Check sheet for the modelled part. Datum: model origin and axes. Units: mm. A direction names the side the tool comes from. Round coordinates to 2 decimals unless told otherwise and drop trailing zeros. Loops run counter-clockwise (first coordinate to the right, second up) from the corner with the lowest first, then second, coordinate; pieces in that order, holes last. Notation, with made-up numbers: (-28.5, 63) - (-16.5, 63) arc R17 ccw to (-16.5, 90) - close; hole circle Ø1 at (6, 21.5). An arc over 180 degrees is marked (long way). Answer in a Markdown table with one row per item. Add a question column.
(1) Mould release check, pull along X, two halves, no side actions. Record for faces 1 (the flat face through (-2, 25.4, 2)), 2 (the flat face through (-244.475, 0, -60)), 3 (the flat face through (-2, -25.4, 2)), 4 (the flat face through (170, -31.75, -55)): +X half, -X half, draft (parallel to the pull), parting line (faces both ways), or undercut.
(2) Access from +Z, -Z, +X, -X, +Y, -Y to the whole of each face (thin tool, end or side, straight path). Record for faces 5 (the flat face through (-15, 0, 0)), 6 (the flat face through (-218, 0, -44.45)), 7 (the flat face through (175, 0, -76.2)), 8 (the flat face through (218, 0, -44.45)), 9 (the flat face through (1, 0, 50.8)).
(3) Cross-section at B-B on z = -20. Enter the section's corners in (x, y), then the cut area to 3 significant figures.
(4) Gauge pin test, flat ends, axial feed: pin 1 (5 mm diameter, centred on y = -16, z = 14.5, fed in from +X); pin 2 (15 mm diameter, centred on x = -8.5, y = 4.5, fed in from -Z); pin 3 (1 mm diameter, centred on y = 17, z = -9.5, fed in from -X). Record the tip position at first contact, or that the pin passes through.
(5) Cross-section at A-A on y = 20. Enter the section's corners in (x, z) (3 decimals).
(6) Cross-section at D-D on y = -6. Enter the section's corners in (x, z) (3 decimals).
(7) Thickness scan on line 1 along Z through (x, y) = (203, 20.5); line 2 along Y through (x, z) = (-83, -32). Record the ranges inside material, lowest first.
(8) Cross-section at C-C on x = 204. Enter the section's corners in (y, z).
from build123d import *

# Parameters (mm, degrees)
F1_DEPTH     = 25.4
F2_DEPTH     = 31.75
F3_T4_DEPTH  = 86.0090909091
F3_T9_DEPTH  = 86.0090909091
F3_T14_DEPTH = 86.0090909091
F3_T19_DEPTH = 86.0090909091
F3_T21_DEPTH = 93.5090909091


# Not quite as in the source:
# - a fillet or chamfer that OpenCascade refuses, or shapes differently, is made with other operations: its cross-section is extruded or revolved along the edge and cut away or added


with BuildPart() as f1:
    # F0 (on Front) → F1 (new body, symmetric)
    with BuildSketch(Plane.XZ):
        with BuildLine():
            Line((-107.95, -76.2), (-63.0464285714, 0))
            Line((-63.0464285714, 0), (0, 0))
            Line((0, 0), (0, 9.525))
            ThreePointArc((0, 9.525), (8.6950956004, 6.9319779212), (14.5496778315, 0))
            Line((14.5496778315, 0), (63.0464285714, 0))
            Line((63.0464285714, 0), (107.95, -76.2))
            Line((107.95, -76.2), (120.65, -76.2))
            Line((120.65, -76.2), (120.65, 2.3090909091))
            Line((120.65, 2.3090909091), (92.075, 50.8))
            Line((92.075, 50.8), (-92.075, 50.8))
            Line((-92.075, 50.8), (-120.65, 2.3090909091))
            Line((-120.65, 2.3090909091), (-120.65, -76.2))
            Line((-120.65, -76.2), (-107.95, -76.2))
        make_face()
        with BuildLine():
            Line((0, 9.525), (0, 0))
            Line((0, 0), (14.5496778315, 0))
            ThreePointArc((14.5496778315, 0), (8.6950956004, 6.9319779212), (0, 9.525))
        make_face()
    extrude(amount=F1_DEPTH, both=True)

    # F0 (on Front) → F2 (join, symmetric)
    with BuildSketch(Plane.XZ):
        with BuildLine():
            Line((-244.475, -76.2), (-120.65, -76.2))
            Line((-120.65, -76.2), (-120.65, 2.3090909091))
            Line((-120.65, 2.3090909091), (-126.0980906593, -6.9361538462))
            ThreePointArc((-126.0980906593, -6.9361538462), (-153.9415343258, -34.4101274299), (-191.7473214286, -44.45))
            Line((-191.7473214286, -44.45), (-244.475, -44.45))
            Line((-244.475, -44.45), (-244.475, -76.2))
        make_face()
        with BuildLine():
            Line((120.65, 2.3090909091), (120.65, -76.2))
            Line((120.65, -76.2), (244.475, -76.2))
            Line((244.475, -76.2), (244.475, -44.45))
            Line((244.475, -44.45), (191.7473214286, -44.45))
            ThreePointArc((191.7473214286, -44.45), (153.9415343258, -34.4101274299), (126.0980906593, -6.9361538462))
            Line((126.0980906593, -6.9361538462), (120.65, 2.3090909091))
        make_face()
    extrude(amount=F2_DEPTH, both=True)

    # F3: fillet of radius 3 on 8 edges, made by hand


with BuildPart() as f3_tool2:
    # F3_s3 → F3_t4 (new body)
    with BuildSketch(Plane.XY.offset(9.8090909091)):
        with BuildLine():
            ThreePointArc((-120.65, -28.4), (-119.7713203436, -26.2786796564), (-117.65, -25.4))
            Line((-117.65, -25.4), (-120.65, -25.4))
            Line((-120.65, -25.4), (-120.65, -28.4))
        make_face()
    extrude(amount=-F3_T4_DEPTH)

    split(bisect_by=Plane(origin=(-90.5622721893, 0, 53.3670532544), x_dir=(0, 1, 0), z_dir=(0.8615384615, 0, -0.5076923077)), keep=Keep.TOP)


with BuildPart() as f1_1:
    add(f1.part)

    # F3_t1: union F3_tool2
    add(f3_tool2.part)


with BuildPart() as f3_tool7:
    # F3_s8 → F3_t9 (new body)
    with BuildSketch(Plane.XY.offset(9.8090909091)):
        with BuildLine():
            ThreePointArc((-120.65, 28.4), (-119.7713203436, 26.2786796564), (-117.65, 25.4))
            Line((-117.65, 25.4), (-120.65, 25.4))
            Line((-120.65, 25.4), (-120.65, 28.4))
        make_face()
    extrude(amount=-F3_T9_DEPTH)

    split(bisect_by=Plane(origin=(-90.5622721893, 0, 53.3670532544), x_dir=(0, 1, 0), z_dir=(0.8615384615, 0, -0.5076923077)), keep=Keep.TOP)


with BuildPart() as f1_2:
    add(f1_1.part)

    # F3_t6: union F3_tool7
    add(f3_tool7.part)


with BuildPart() as f3_tool12:
    # F3_s13 → F3_t14 (new body)
    with BuildSketch(Plane.XY.offset(-76.2)):
        with BuildLine():
            ThreePointArc((117.65, 25.4), (119.7713203436, 26.2786796564), (120.65, 28.4))
            Line((120.65, 28.4), (120.65, 25.4))
            Line((120.65, 25.4), (117.65, 25.4))
        make_face()
    extrude(amount=F3_T14_DEPTH)

    split(bisect_by=Plane(origin=(90.5622721893, 0, 53.3670532544), x_dir=(0, 1, 0), z_dir=(-0.8615384615, 0, -0.5076923077)), keep=Keep.TOP)


with BuildPart() as f1_3:
    add(f1_2.part)

    # F3_t11: union F3_tool12
    add(f3_tool12.part)


with BuildPart() as f3_tool17:
    # F3_s18 → F3_t19 (new body)
    with BuildSketch(Plane.XY.offset(-76.2)):
        with BuildLine():
            ThreePointArc((117.65, -25.4), (119.7713203436, -26.2786796564), (120.65, -28.4))
            Line((120.65, -28.4), (120.65, -25.4))
            Line((120.65, -25.4), (117.65, -25.4))
        make_face()
    extrude(amount=F3_T19_DEPTH)

    split(bisect_by=Plane(origin=(90.5622721893, 0, 53.3670532544), x_dir=(0, 1, 0), z_dir=(-0.8615384615, 0, -0.5076923077)), keep=Keep.TOP)


with BuildPart() as f1_4:
    add(f1_3.part)

    # F3_t16: union F3_tool17
    add(f3_tool17.part)

    # F3_s22 → F3_t21 (cut)
    with BuildSketch(Plane.XY.offset(-83.7)):
        with BuildLine():
            ThreePointArc((-120.65, -28.75), (-121.5286796564, -30.8713203436), (-123.65, -31.75))
            Line((-123.65, -31.75), (-120.65, -31.75))
            Line((-120.65, -31.75), (-120.65, -28.75))
        make_face()
        with BuildLine():
            ThreePointArc((-123.65, 31.75), (-121.5286796564, 30.8713203436), (-120.65, 28.75))
            Line((-120.65, 28.75), (-120.65, 31.75))
            Line((-120.65, 31.75), (-123.65, 31.75))
        make_face()
        with BuildLine():
            ThreePointArc((120.65, 28.75), (121.5286796564, 30.8713203436), (123.65, 31.75))
            Line((123.65, 31.75), (120.65, 31.75))
            Line((120.65, 31.75), (120.65, 28.75))
        make_face()
        with BuildLine():
            ThreePointArc((123.65, -31.75), (121.5286796564, -30.8713203436), (120.65, -28.75))
            Line((120.65, -28.75), (120.65, -31.75))
            Line((120.65, -31.75), (123.65, -31.75))
        make_face()
    extrude(amount=F3_T21_DEPTH, mode=Mode.SUBTRACT)

    # F0 (on Front) → F4 (revolve, cut)
    with BuildSketch(Plane.XZ):
        with BuildLine():
            Line((0, 9.525), (0, 0))
            Line((0, 0), (14.5496778315, 0))
            ThreePointArc((14.5496778315, 0), (8.6950956004, 6.9319779212), (0, 9.525))
        make_face()
    revolve(axis=Axis((0, 0, 4.7625), (0, 0, -1)), mode=Mode.SUBTRACT)


solid = f1_4.part
Answers:
| question | item | result |
|---|---|---|
| 1 | face 1 | undercut |
| 1 | face 2 | -X half |
| 1 | face 3 | undercut |
| 1 | face 4 | draft |
| 2 | face 5 | -Z, +Y, -Y |
| 2 | face 6 | +Z, -X, +Y, -Y |
| 2 | face 7 | -Z, +X, -X, +Y, -Y |
| 2 | face 8 | +Z, +X, +Y, -Y |
| 2 | face 9 | +Z, +X, -X, +Y, -Y |
| 3 | outline | (-135.82, -31.75) - (-123.65, -31.75) arc R3 ccw to (-120.65, -28.75) - (-120.65, -28.4) arc R3 cw to (-117.65, -25.4) - (-74.83, -25.4) - (-74.83, 25.4) - (-117.65, 25.4) arc R3 cw to (-120.65, 28.4) - (-120.65, 28.75) arc R3 ccw to (-123.65, 31.75) - (-135.82, 31.75) - close; (74.83, -25.4) - (117.65, -25.4) arc R3 cw to (120.65, -28.4) - (120.65, -28.75) arc R3 ccw to (123.65, -31.75) - (135.82, -31.75) - (135.82, 31.75) - (123.65, 31.75) arc R3 ccw to (120.65, 28.75) - (120.65, 28.4) arc R3 cw to (117.65, 25.4) - (74.83, 25.4) - close |
| 3 | area | 6,580 mm^2 |
| 4 | pin 1 | stops at x = 114.94 |
| 4 | pin 2 | stops at z = 0 |
| 4 | pin 3 | stops at x = -128 |
| 5 | outline | (-244.475, -76.2) - (-107.95, -76.2) - (-63.046, 0) - (63.046, 0) - (107.95, -76.2) - (244.475, -76.2) - (244.475, -44.45) - (191.747, -44.45) arc R76.2 cw to (126.098, -6.936) - (92.075, 50.8) - (-92.075, 50.8) - (-126.098, -6.936) arc R76.2 cw to (-191.747, -44.45) - (-244.475, -44.45) - close |
| 6 | outline | (-244.475, -76.2) - (-107.95, -76.2) - (-63.046, 0) - (-13.255, 0) arc R14.697 cw to (13.255, 0) - (63.046, 0) - (107.95, -76.2) - (244.475, -76.2) - (244.475, -44.45) - (191.747, -44.45) arc R76.2 cw to (126.098, -6.936) - (92.075, 50.8) - (-92.075, 50.8) - (-126.098, -6.936) arc R76.2 cw to (-191.747, -44.45) - (-244.475, -44.45) - close |
| 7 | line 1 | z = -76.2 to -44.45 |
| 7 | line 2 | y = -25.4 to 25.4 |
| 8 | outline | (-31.75, -76.2) - (31.75, -76.2) - (31.75, -44.45) - (-31.75, -44.45) - close |
